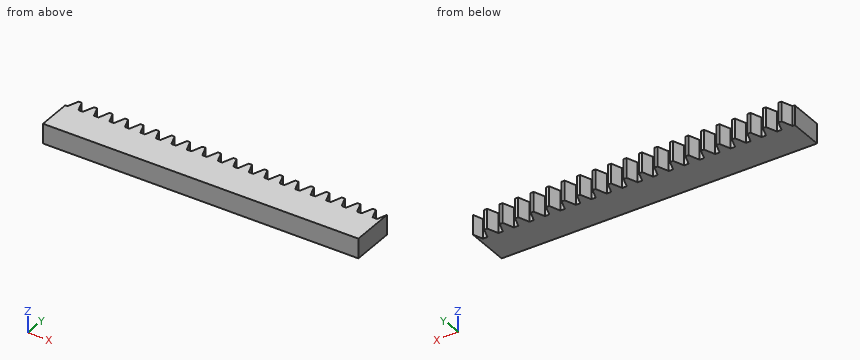
```python
from build123d import *

# Parameters (mm, degrees)
BLANKSKE_W        = 50.8
BLANKSKE_H        = 7.14375
BLANK_DEPTH       = 3.175
TOOTHCUTSIM_DEPTH = 52.397994018
TEETHCUTS_COUNT   = 21
TEETHCUTS_PITCH   = 2.493639166


with BuildPart() as part:
    # BlankSke → Blank (new body)
    with BuildSketch(Plane.XY):
        with Locations((25.4, 3.571875)):
            Rectangle(BLANKSKE_W, BLANKSKE_H)
    extrude(amount=-BLANK_DEPTH)

    # TooCutSkeSim → ToothCutSim (cut, through all)
    with BuildSketch(Plane.XY):
        Polygon((0.362072143, 5.3975), (-0.362072143, 5.3975), (-1.006900009, 7.16915), (1.006900009, 7.16915), align=None)
    toothcutsim = extrude(amount=-TOOTHCUTSIM_DEPTH, mode=Mode.SUBTRACT)

    # TeethCuts: ToothCutSim ×21
    with Locations(*[(i * TEETHCUTS_PITCH, 0, 0) for i in range(1, TEETHCUTS_COUNT)]):
        add(toothcutsim, mode=Mode.SUBTRACT)


solid = part.part
```
The model under review builds one solid part; all positions refer to its coordinate system, in mm. Coordinates: 2 decimals unless noted, no trailing zeros. Answer in a Markdown table with one row per item. Add a question column.
Q1. To check wall thickness, follow line 1 along Y through (x, z) = (22.5, -2.65). State the ranges of the line that lie inside material, in increasing order. Write a range as from..to.
Q2. Clearance check with flat-ended pins moving along their axes: pin 1 (4 mm diameter, centred on x = 16, y = 3.5, fed in from +Z); pin 2 (0.6 mm diameter, centred on x = 5, z = -2, fed in from +Y). State where each tip first meets the part, or that it passes through.
Q3. Consider section A-A on y = 6. Give the number of separate pieces and of enclosed holes in the cut face, then the cut area to 3 significant figures.
Answers below:
| question | item | result |
|---|---|---|
| 1 | line 1 | 0..5.4 |
| 2 | pin 1 | z = 0 |
| 2 | pin 2 | y = 5.4 |
| 3 | separate pieces | 21 |
| 3 | enclosed holes | 0 |
| 3 | area | 85.6 mm² |
